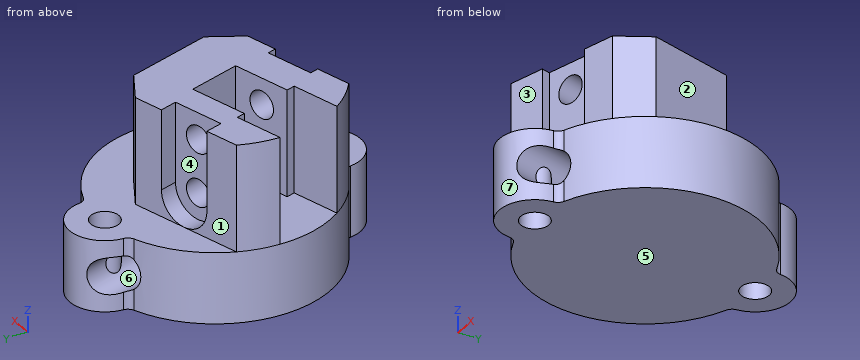
```python
from build123d import *

# Parameters (mm, degrees)
SKETCH1_R               = 1.6
BOSS_EXTRUDE1_DEPTH     = 8.00600005
CUT_EXTRUDE1_DEPTH      = 23.553404107
CUT_EXTRUDE1_DEPTH_BACK = 23.553404107
SKETCH3_R               = 2.1
BOSS_EXTRUDE2_DEPTH     = 12
CHAMFER1_SIZE           = 3
CUT_EXTRUDE4_DEPTH      = 35.916819883
CUT_EXTRUDE4_DEPTH_BACK = 35.916819883
SKETCH7_R               = 1.55
CUT_EXTRUDE5_DEPTH      = 2
CUT_EXTRUDE5_DEPTH_BACK = 1
CUT_EXTRUDE6_DEPTH      = 2


with BuildPart() as part:
    # Sketch1 → Boss-Extrude1 (new body)
    with BuildSketch(Plane.XY):
        with BuildLine():
            ThreePointArc((4.62089851, -12.151020408), (13, 0), (4.62089851, 12.151020408))
            ThreePointArc((4.62089851, 12.151020408), (4.181690754, 12.478661471), (3.981081793, 12.988571429))
            ThreePointArc((3.981081793, 12.988571429), (0, 16.6), (-3.981081793, 12.988571429))
            ThreePointArc((-3.981081793, 12.988571429), (-4.181690754, 12.478661471), (-4.62089851, 12.151020408))
            ThreePointArc((-4.62089851, 12.151020408), (-13, 0), (-4.62089851, -12.151020408))
            ThreePointArc((-4.62089851, -12.151020408), (-4.181690754, -12.478661471), (-3.981081793, -12.988571429))
            ThreePointArc((-3.981081793, -12.988571429), (0, -16.6), (3.981081793, -12.988571429))
            ThreePointArc((3.981081793, -12.988571429), (4.181690754, -12.478661471), (4.62089851, -12.151020408))
        make_face()
        with Locations((0, 12.6)):
            Circle(SKETCH1_R, mode=Mode.SUBTRACT)
        with Locations((0, -12.6)):
            Circle(SKETCH1_R, mode=Mode.SUBTRACT)
    extrude(amount=BOSS_EXTRUDE1_DEPTH)

    # Sketch3 → Cut-Extrude1 (cut, two sides: drawn at the far end of the back side and taken through both)
    with BuildSketch(Plane(origin=(0, 0, 0), x_dir=(0, 0, 1), z_dir=(-0.25881904510252135, 0.9659258262890681, 0)).offset(-CUT_EXTRUDE1_DEPTH_BACK)):
        with Locations(Location((4.003000025, 0, 0), (0, 0, 218.89324433))):
            Circle(SKETCH3_R)
    extrude(amount=CUT_EXTRUDE1_DEPTH + CUT_EXTRUDE1_DEPTH_BACK, mode=Mode.SUBTRACT)

    # Sketch6 → Boss-Extrude2 (add)
    with BuildSketch(Plane.XY.offset(8.00600005)):
        with BuildLine():
            Line((-7.827242025, -10.379512623), (7.962699901, -6.148610435))
            Line((7.962699901, -6.148610435), (3.82159518, 9.306202785))
            Line((3.82159518, 9.306202785), (-11.968346746, 5.075300598))
            ThreePointArc((-11.968346746, 5.075300598), (-12.66343786, 2.938935449), (-12.9803337, 0.714798598))
            Line((-12.9803337, 0.714798598), (-7.519920169, 2.177911994))
            Line((-7.519920169, 2.177911994), (-7.261101124, 1.211986168))
            Line((-7.261101124, 1.211986168), (-0.692805505, 2.971955675))
            Line((-0.692805505, 2.971955675), (0.88599067, -2.920191866))
            Line((0.88599067, -2.920191866), (-5.682304949, -4.680161372))
            Line((-5.682304949, -4.680161372), (-5.423485903, -5.646087199))
            Line((-5.423485903, -5.646087199), (-10.883899435, -7.109200595))
            ThreePointArc((-10.883899435, -7.109200595), (-9.497391161, -8.876911689), (-7.827242025, -10.379512623))
        make_face()
    extrude(amount=BOSS_EXTRUDE2_DEPTH)

    # Chamfer1
    chamfer1_edges = [part.edges().sort_by_distance(p)[0] for p in [
        (7.962699901, -6.148610435, 14.00600005),
        (3.82159518, 9.306202785, 14.00600005),
    ]]
    chamfer(chamfer1_edges, length=CHAMFER1_SIZE)

    # Sketch7 → Cut-Extrude4 (cut, two sides: drawn at the far end of the back side and taken through both)
    with BuildSketch(Plane(origin=(-2.070552361, 7.72740661, 0), x_dir=(0.9659258262890701, 0.2588190451025142, 0), z_dir=(-0.2588190451025142, 0.9659258262890701, 0)).offset(-CUT_EXTRUDE4_DEPTH_BACK)):
        with Locations(Location((-3.346950766, -17.00600005, 0), (0, 0, 180))):
            Circle(SKETCH7_R)
        with Locations(Location((-3.346950766, -11.00600005, 0), (0, 0, 180))):
            Circle(SKETCH7_R)
    extrude(amount=CUT_EXTRUDE4_DEPTH + CUT_EXTRUDE4_DEPTH_BACK, mode=Mode.SUBTRACT)

    # Sketch8 → Cut-Extrude5 (cut, two sides: drawn at the far end of the back side and taken through both)
    with BuildSketch(Plane(origin=(2.070552361, -7.72740661, 0), x_dir=(0.9659258262890699, 0.25881904510251513, 0), z_dir=(0.2588190451025151, -0.9659258262890698, 0)).offset(-CUT_EXTRUDE5_DEPTH_BACK)):
        Polygon((-6.146950766, 12.622580803), (-6.146950766, 20.00600005), (-0.546950766, 20.00600005), (-0.546950766, 12.622580803), (-0.546950766, 9.389419296), (-3.346950766, 7.772838542), (-6.146950766, 9.389419296), align=None)
    extrude(amount=CUT_EXTRUDE5_DEPTH + CUT_EXTRUDE5_DEPTH_BACK, mode=Mode.SUBTRACT)

    # Sketch9 → Cut-Extrude6 (cut)
    with BuildSketch(Plane(origin=(-2.070552361, 7.72740661, 0), x_dir=(0.9659258262890701, 0.2588190451025142, 0), z_dir=(-0.2588190451025142, 0.9659258262890701, 0))):
        with BuildLine():
            Line((-6.346950766, -20.00600005), (-6.346950766, -11.00600005))
            ThreePointArc((-6.346950766, -11.00600005), (-3.346950766, -8.00600005), (-0.346950766, -11.00600005))
            Line((-0.346950766, -11.00600005), (-0.346950766, -20.00600005))
            Line((-0.346950766, -20.00600005), (-6.346950766, -20.00600005))
        make_face()
    extrude(amount=-CUT_EXTRUDE6_DEPTH, mode=Mode.SUBTRACT)


solid = part.part
```
CAD build for the part. Positions are in the model's coordinates, mm. Face numbers are marked on the shaded views. A direction names the side the tool comes from. Coordinates: 2 decimals unless noted, no trailing zeros. Loops run counter-clockwise (first coordinate to the right, second up) from the corner with the lowest first, then second, coordinate; pieces in that order, holes last. Notation, with made-up numbers: (-8.5, 85.25) - (26.5, 85.25) arc R25 ccw to (26.5, 104.25) - close; hole circle Ø9 at (10, 25.5). An arc over 180 degrees is marked (long way). Return JSON: item names as keys, results as strings.
1. Band-saw the part on A-A (z = 13.75). Give the cut face in (x, y).
Result:
{"outline": "(-12.98, 0.71) - (-7.52, 2.18) - (-7.26, 1.21) - (-0.69, 2.97) - (0.89, -2.92) - (-5.68, -4.68) - (-5.42, -5.65) - (-10.88, -7.11) arc R13 ccw to (-7.83, -10.38) - (-3.87, -9.32) - (-4.13, -8.35) - (1.28, -6.9) - (1.54, -7.87) - (5.06, -6.93) - (7.19, -3.25) - (4.6, 6.41) - (0.92, 8.53) - (-2.41, 7.64) - (-1.89, 5.71) - (-7.68, 4.15) - (-8.2, 6.08) - (-11.97, 5.08) arc R13 ccw to start"}
2. Probe L1, parallel to Y at x = 0, z = 1.75; L2, parallel to Y at x = -1, z = 7; L3, parallel to X at y = 12.6, z = 5.5. List the from-to ranges inside material, lowest first. Write a range as from..to.
Result:
{"L1": "y = -16.6..-14.2, -11..11, 14.2..16.6", "L2": "y = -16.47..-13.85, -11.35..11.35, 13.85..16.47", "L3": "x = -1.85..-1.6, 1.6..4.1"}
3. Drop flat-ended pins along their axis: pin 1 (1 mm diameter, centred on x = 10, z = 2.5, fed in from +Y); pin 2 (1 mm diameter, centred on y = -12, z = 5, fed in from +X); pin 3 (3 mm diameter, centred on x = 0, y = 12.6, fed in from +Z); pin 4 (3 mm diameter, centred on x = 3.5, z = 5.5, fed in from +Y). Give the stop position or say it passes through.
Result:
{"pin 1": "stops at y = 8.87", "pin 2": "stops at x = 6.06", "pin 3": "passes through", "pin 4": "stops at y = 16.06"}
4. Band-saw the part on B-B (y = -12.6). State how many separate pieces and enclosed holes the cut face has, and give its area (3 significant figures).
Result:
{"separate pieces": "3", "enclosed holes": "0", "area": "30.6 mm2"}
5. Mould opens along Y. For the marked faces 4, 5, 6 and 7 say: released by +Y, released by -Y, zero draft, split by the parting line, or undercut.
Result:
{"face 4": "undercut", "face 5": "zero draft", "face 6": "undercut", "face 7": "released by -Y"}
6. 3-axis set-ups, long thin cutter, end or side, ignore diameter. For the marked faces 1, 2 and 3: which of +Z, -Z, +X, -X, +Y, -Y reach the whole face in a straight line?
Result:
{"face 1": "+Z, -X, +Y", "face 2": "+Z, +X, +Y", "face 3": "+Z, +X, -Y"}
